For this review, take the finished solid that the model builds, in its own axes (mm). Face numbers are marked on the shaded views. A direction names the side the tool comes from. Give positions to 0.01 mm unless a question says otherwise; leave off trailing zeros. Order: outer loops, then holes, each group sorted by start corner. A loop starts at its lowest first (then second) coordinate and runs counter-clockwise, first axis right, second up. Notation, with made-up numbers: (83.25, -20.75) -> (130.25, -20.75) arc R24 ccw to (130.25, -4.75) -> close; hole circle Ø6 at (-30, 1.25). An arc over 180 degrees is marked (long way). Return JSON: item names as keys, results as strings. Group by question number.
1) For the marked faces 1 and 2, list the 3-axis set-ups (+Z, -Z, +X, -X, +Y, -Y) from which the entire face can be reached by the end or side of a thin tool; tool diameter is ignored.
2) To check wall thickness, follow line 1 along Z through (x, y) = (27, 0); line 2 along Y through (x, z) = (37, 34); line 3 along X through (y, z) = (28.5, 25). State the ranges of each line that lie inside material, in increasing order.
3) Add section D-D (y = -39.5). Give the boundary of the cut face in (x, z).
4) Insertion check: P1, Ø6, axis at x = 39, y = 19.5, coming from the -Z side; P2, Ø10, axis at y = 11, z = 25.5, coming from the +X side; P3, Ø5, axis at x = 39, y = -7.5, coming from the +Z side; P4, Ø2, axis at x = 41.5, z = 56, coming from the +Y side. Each pin has a flat end and moves straight along its axis. Give the tip position at first contact, or say it passes through.
5) The part is to be moulded in two halves that separate along Z. For the marked faces 3, 4, 5 and 6, say which applies: released by +Z, released by -Z, zero draft, split by the parting line, or undercut.
6) Add section A-A (y = 0). Give the boundary of the cut face in (x, z).
7) Add section B-B (z = 34.5). Give the boundary of the cut face in (x, y), then the cut area to 3 significant figures.
8) Add section C-C (x = 21). Give the boundary of the cut face in (y, z) (3 decimals).
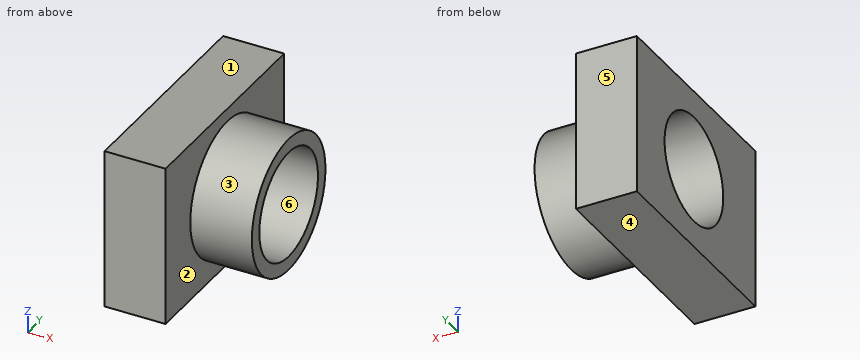
from build123d import *

# Parameters (mm, degrees)
F0_W     = 25.1680966467
F0_H     = 89.8744724691
F1_DEPTH = 66.294
F2_R     = 27.8892037899
F3_DEPTH = 25.4
F5_D     = 44.45


with BuildPart() as f1:
    # F0 (on Top) → F1 (new body)
    with BuildSketch(Plane.XY):
        with Locations((12.5840483233, -1.6976874322)):
            Rectangle(F0_W, F0_H)
    extrude(amount=F1_DEPTH)

    # F2 (on face) → F3 (join)
    with BuildSketch(Plane.YZ.offset(25.1680966467)):
        with Locations((0, 33.0868437886)):
            Circle(F2_R)
    extrude(amount=F3_DEPTH)

    # F5 (through all)
    with Locations(Plane.YZ.offset(50.5680966467)):
        with Locations((0, 33.0868437886)):
            Hole(F5_D / 2)


solid = f1.part
Evaluation:
{
 "1": {"face 1": "+Z, +X, -X, +Y, -Y", "face 2": "+X"},
 "2": {"line 1": "5.2 to 10.86, 55.31 to 60.98", "line 2": "-27.87 to -22.21, 22.21 to 27.87", "line 3": "0 to 25.17"},
 "3": {"outline": "(0, 0) -> (25.17, 0) -> (25.17, 66.29) -> (0, 66.29) -> close"},
 "4": {"P1": "z = 10.6", "P2": "through", "P3": "z = 60.52", "P4": "y = 17.25"},
 "5": {"face 3": "split by the parting line", "face 4": "released by -Z", "face 5": "zero draft", "face 6": "undercut"},
 "6": {"outline": "(0, 0) -> (25.17, 0) -> (25.17, 5.2) -> (50.57, 5.2) -> (50.57, 10.86) -> (0, 10.86) -> close; (0, 55.31) -> (50.57, 55.31) -> (50.57, 60.98) -> (25.17, 60.98) -> (25.17, 66.29) -> (0, 66.29) -> close"},
 "7": {"outline": "(0, -46.63) -> (25.17, -46.63) -> (25.17, -27.85) -> (50.57, -27.85) -> (50.57, -22.18) -> (0, -22.18) -> close; (0, 22.18) -> (50.57, 22.18) -> (50.57, 27.85) -> (25.17, 27.85) -> (25.17, 43.24) -> (0, 43.24) -> close", "area": "1,430 mm^2"},
 "8": {"outline": "(-46.635, 0) -> (43.24, 0) -> (43.24, 66.294) -> (-46.635, 66.294) -> close; hole circle Ø44.45 at (0, 33.087)"}
}
